The model under review builds one solid part; all positions refer to its coordinate system, in mm. A direction names the side the tool comes from. Round coordinates to 2 decimals unless told otherwise and drop trailing zeros. Write each loop counter-clockwise with the first axis right and the second up, starting at its lowest first coordinate (ties: lowest second). Pieces come first, ordered by that corner, then holes.
Item 1: Machinability: for faces 1 (the face through (-1, 13, 2)), 2 (the face through (0, 1.75, 4)), which of the approach directions +Z, -Z, +X, -X, +Y, -Y give a long, thin tool a straight path to every point of the face, cutting with its end or side? Answer none if there is none.
Item 2: Add section D-D (y = 9.75). Give the boundary of the cut face in (x, z) (3 decimals), plus the area to 3 significant figures.
Item 3: Clearance check with flat-ended pins moving along their axes: pin 1 Ø4 at (x, y) = (1, 1.5) entering from -Z; pin 2 Ø3 at (y, z) = (6.5, -2) entering from +X; pin 3 Ø4 at (y, z) = (1.5, 2.5) entering from -X. State where each tip first meets the part, or that it passes through.
Item 4: Add section A-A (z = 0). Give the boundary of the cut face in (x, y) (3 decimals), plus the area to 4 significant figures.
Item 5: To check wall thickness, follow L1, parallel to Y at x = -2.5, z = -2.5 (3 decimals); L2, parallel to Z at x = 0, y = 7.25 (3 decimals); L3, parallel to X at y = 9.5, z = 0 (3 decimals). State the ranges of each line that lie inside material, in increasing order.
Item 6: Draft analysis for pull direction X (two halves, no side actions). For faces 3 (the face through (1, 0, 2)), 4 (the face through (3.233, 2.798, 1.341)), 5 (the face through (-1.873, 6.591, -0.082)), state which applies: +X half, -X half, draft (parallel to the pull), parting line (faces both ways), or undercut.
Item 7: Add section C-C (z = -3.75). Give the boundary of the cut face in (x, y) (3 decimals), plus the area to 3 significant figures.
Item 8: Add section B-B (x = 0). Give the boundary of the cut face in (y, z) (3 decimals), plus the area to 4 significant figures.
```python
from build123d import *

# Parameters (mm, degrees)
SKETCH2_R               = 1.875
CUT_EXTRUDE1_DEPTH      = 1
CUT_EXTRUDE1_DEPTH_BACK = 14


with BuildPart() as part:
    # Sketch1 → Revolve1 (revolve)
    with BuildSketch(Plane.XY):
        Polygon((0, 0), (0, 13), (4.5, 13), (4.5, 11.25), (3.5, 11.25), (3.5, 9.125), (4.5, 9.125), (4.5, 3.875), (3.5, 3.875), (3.5, 1.75), (4.5, 1.75), (4.5, 0), align=None)
    revolve(axis=Axis((0, 0, 0), (0, 1, 0)))

    # Sketch2 → Cut-Extrude1 (cut, two sides)
    with BuildSketch(Plane(origin=(0, 13, 0), x_dir=(1, 0, 0), z_dir=(0, 1, 0))) as cut_extrude1_sk:
        Circle(SKETCH2_R)
    extrude(amount=CUT_EXTRUDE1_DEPTH, mode=Mode.SUBTRACT)
    extrude(cut_extrude1_sk.sketch, amount=-CUT_EXTRUDE1_DEPTH_BACK, mode=Mode.SUBTRACT)


solid = part.part
```
Numbers:
1. face 1: +Z, -Z, +X, -X, +Y
1. face 2: none
2. outline: circle Ø7 at (0, 0); hole circle Ø3.75 at (0, 0)
2. area: 27.4 mm2
3. pin 1: stops at z = -4.5
3. pin 2: stops at x = 4.47
3. pin 3: stops at x = -4.47
4. outline: (-4.5, 0) - (-1.875, 0) - (-1.875, 13) - (-4.5, 13) - (-4.5, 11.25) - (-3.5, 11.25) - (-3.5, 9.125) - (-4.5, 9.125) - (-4.5, 3.875) - (-3.5, 3.875) - (-3.5, 1.75) - (-4.5, 1.75) - close; (1.875, 0) - (4.5, 0) - (4.5, 1.75) - (3.5, 1.75) - (3.5, 3.875) - (4.5, 3.875) - (4.5, 9.125) - (3.5, 9.125) - (3.5, 11.25) - (4.5, 11.25) - (4.5, 13) - (1.875, 13) - close
4. area: 59.75 mm2
5. L1: y = 0 to 1.75, 3.875 to 9.125, 11.25 to 13
5. L2: z = -4.5 to -1.875, 1.875 to 4.5
5. L3: x = -3.5 to -1.875, 1.875 to 3.5
6. face 3: draft
6. face 4: parting line
6. face 5: undercut
7. outline: (-2.487, 0) - (2.487, 0) - (2.487, 1.75) - (-2.487, 1.75) - close; (-2.487, 3.875) - (2.487, 3.875) - (2.487, 9.125) - (-2.487, 9.125) - close; (-2.487, 11.25) - (2.487, 11.25) - (2.487, 13) - (-2.487, 13) - close
7. area: 43.5 mm2
8. outline: (0, -4.5) - (1.75, -4.5) - (1.75, -3.5) - (3.875, -3.5) - (3.875, -4.5) - (9.125, -4.5) - (9.125, -3.5) - (11.25, -3.5) - (11.25, -4.5) - (13, -4.5) - (13, -1.875) - (0, -1.875) - close; (0, 1.875) - (13, 1.875) - (13, 4.5) - (11.25, 4.5) - (11.25, 3.5) - (9.125, 3.5) - (9.125, 4.5) - (3.875, 4.5) - (3.875, 3.5) - (1.75, 3.5) - (1.75, 4.5) - (0, 4.5) - close
8. area: 59.75 mm2
